Verification items for the finished model (mm, model axes). A direction names the side the tool comes from. Give positions to 0.01 mm unless a question says otherwise; leave off trailing zeros. Write each loop counter-clockwise with the first axis right and the second up, starting at its lowest first coordinate (ties: lowest second). Pieces come first, ordered by that corner, then holes. Notation, with made-up numbers: M 74.25,14.25 L 106.25,14.25 A28 ccw 106.25,45.25 Z; hole C -2.75,-37 d11. An arc over 180 degrees is marked long. Answer as a JSON object with one key per item and string values.
```python
from build123d import *

# Parameters (mm, degrees)
F1_DEPTH       = 3
F2_SIZE        = 0.5
F4_D           = 3.4
F4_CSINK_D     = 6.3
F4_CSINK_ANGLE = 90
F5_R           = 8
F6_DEPTH       = 13
F7_R           = 5
F8_DEPTH       = 14
F9_R           = 4.5
F10_DEPTH      = 16
F11_SIZE       = 1.5
F12_SIZE       = 0.49999


# Not quite as in the source:
# - a fillet or chamfer is up to 0.001 mm smaller than in the source, because OpenCascade refuses the exact size


with BuildPart() as f1:
    # F0 (on Top) → F1 (new body)
    with BuildSketch(Plane.XY):
        with BuildLine():
            Line((11.1242977306, 8.5), (-11.1242977306, 8.5))
            ThreePointArc((-11.1242977306, 8.5), (-14, 0), (-11.1242977306, -8.5))
            Line((-11.1242977306, -8.5), (11.1242977306, -8.5))
            ThreePointArc((11.1242977306, -8.5), (14, 0), (11.1242977306, 8.5))
        make_face()
    extrude(amount=F1_DEPTH)

    # F2
    f2_edges = [f1.edges().sort_by_distance(p)[0] for p in [
        (0, -8.5, 3),
        (14, 0, 3),
        (0, 8.5, 3),
        (-14, 0, 3),
        (0, -8.5, 0),
        (14, 0, 0),
        (0, 8.5, 0),
        (-14, 0, 0),
    ]]
    chamfer(f2_edges, length=F2_SIZE)

    # F4 (through all)
    with Locations(Plane.XY.offset(3)):
        with Locations((-10, 0), (10, 0)):
            CounterSinkHole(F4_D / 2, F4_CSINK_D / 2, counter_sink_angle=F4_CSINK_ANGLE)

    # F5 (on face) → F6 (join)
    with BuildSketch(Plane(origin=(0, 0, 0), x_dir=(1, 0, 0), z_dir=(0, 0, -1))):
        Circle(F5_R)
    extrude(amount=F6_DEPTH)

    # F7 (on face) → F8 (join)
    with BuildSketch(Plane(origin=(0, 0, -13), x_dir=(1, 0, 0), z_dir=(0, 0, -1))):
        Circle(F7_R)
    extrude(amount=F8_DEPTH)

    # F9 (on face) → F10 (join)
    with BuildSketch(Plane(origin=(0, 0, -27), x_dir=(1, 0, 0), z_dir=(0, 0, -1))):
        Circle(F9_R)
    extrude(amount=F10_DEPTH)

    # F11
    f11_edges = [f1.edges().sort_by_distance(p)[0] for p in [
        (-4.5, 0, -43),
    ]]
    chamfer(f11_edges, length=F11_SIZE)

    # F12 (size 0.5 in the source; OpenCascade refuses exactly that, so slightly less here)
    f12_edges = [f1.edges().sort_by_distance(p)[0] for p in [
        (-5, 0, -27),
        (-8, 0, -13),
    ]]
    chamfer(f12_edges, length=F12_SIZE)


solid = f1.part
```
1) Go/stop test with flat-tipped pins: pin 1 (3 mm diameter, centred on x = 4.5, y = -1, fed in from -Z); pin 2 (8 mm diameter, centred on y = -4.5, z = -24.5, fed in from +X); pin 3 (1.5 mm diameter, centred on y = 0, z = -30.5, fed in from +X); pin 4 (2 mm diameter, centred on x = 10, y = 0, fed in from +Z). Record where each tip stops, or that it passes through.
Completed:
{"pin 1": "stops at z = -42.89", "pin 2": "stops at x = 4.97", "pin 3": "stops at x = 4.5", "pin 4": "passes through"}
2) Section check D-D on z = -16. Record the boundary of the cut face in (x, y), and give its area (3 significant figures).
Completed:
{"outline": "C 0,0 d10", "area": "78.5 mm2"}
3) Section check C-C on z = -27.5. Record the boundary of the cut face in (x, y), and give its area (3 significant figures).
Completed:
{"outline": "C 0,0 d9", "area": "63.6 mm2"}
4) Thickness scan on L1, parallel to X at y = 0, z = 0.75; L2, parallel to Y at x = -10, z = 0.55; L3, parallel to Z at x = 4.75, y = 4.25. Record the ranges inside material, lowest first.
Completed:
{"L1": "x = -14 to -11.7, -8.3 to 8.3, 11.7 to 14", "L2": "y = -8.5 to -1.7, 1.7 to 8.5", "L3": "z = -13 to 3"}
5) Section check B-B on y = 0. Count the separate pieces of the cut face and the enclosed holes in it, and give its area (3 significant figures).
Completed:
{"separate pieces": "3", "enclosed holes": "0", "area": "548 mm2"}
6) Release check for a two-part mould opening along X. For faces 3 (the face through (8.43, -0.65, 0.76)), 4 (the face through (-13.635, 0.125, 2.865)), 5 (the face through (0, 8.5, 1)), 6 (the face through (-0.59, -4.46, -34.15)) record: pulls with the +X half, pulls with the -X half, needs draft (parallel to the pull), parting line crosses it, or undercut.
Completed:
{"face 3": "undercut", "face 4": "pulls with the -X half", "face 5": "needs draft", "face 6": "parting line crosses it"}
7) Access from +Z, -Z, +X, -X, +Y, -Y to the whole of each face (thin tool, end or side, straight path). Record for faces 1 (the face through (5, 2, -13)), 2 (the face through (0, 0, 3)).
Completed:
{"face 1": "-Z", "face 2": "+Z, +X, -X, +Y, -Y"}
8) Section check A-A on x = 10. Record the boundary of the cut face in (y, z), and give its area (3 significant figures).
Completed:
{"outline": "M -8.5,0.5 L -8,0 L -1.7,0 L -1.7,1.55 L -3.15,3 L -8,3 L -8.5,2.5 Z; M 1.7,0 L 8,0 L 8.5,0.5 L 8.5,2.5 L 8,3 L 3.15,3 L 1.7,1.55 Z", "area": "38.2 mm2"}
